Check sheet for the modelled part. Datum: model origin and axes. Units: mm. Coordinates: 2 decimals unless noted, no trailing zeros. Loops run counter-clockwise (first coordinate to the right, second up) from the corner with the lowest first, then second, coordinate; pieces in that order, holes last. Notation, with made-up numbers: (36.5, 20) - (69.5, 20) arc R17 cw to (69.5, 29) - close; hole circle Ø5 at (37.5, 38). An arc over 180 degrees is marked (long way). Write each question's results on one line, items separated by ' | '. Start each with the question number.
1. Cross-section at B-B (x = 2). Record the cut outline in (y, z).
2. Gauge pin test, flat ends, axial feed: P1, Ø1.5, axis at x = 30.5, y = 5.5, coming from the +Z side; P2, Ø0.9, axis at y = 31.5, z = 1, coming from the -X side. Record the tip position at first contact, or that the pin passes through.
3. Cross-section at A-A (y = 13). Record the cut outline in (x, z).
4. Thickness scan on line 1 (Y direction, x = 12.5, z = 0.5); line 2 (Y direction, x = 11, z = 0.2); line 3 (Y direction, x = 41, z = 1.3). Record the ranges inside material, lowest first. Write a range as [from, to].
```python
from build123d import *

# Parameters (mm, degrees)
F1_DEPTH = 1.524


with BuildPart() as f1:
    # F0 (on Top) → F1 (new body)
    with BuildSketch(Plane.XY):
        with BuildLine():
            ThreePointArc((-10.328003, 23.34511), (-10.546485, 19.972041), (-10.513837, 16.592061))
            Line((-10.513837, 16.592061), (10.397906, 16.369229))
            Line((10.397906, 16.369229), (10.397906, 16.592061))
            ThreePointArc((10.397906, 16.592061), (10.430555, 19.972041), (10.212073, 23.34511))
            ThreePointArc((10.212073, 23.34511), (9.373504, 27.05499), (8.504586, 30.75788))
            Line((8.504586, 30.75788), (8.504586, 31.872794))
            ThreePointArc((8.504586, 31.872794), (9.226054, 34.37206), (9.788919, 36.91175))
            ThreePointArc((9.788919, 36.91175), (9.766765, 38.207065), (9.636335, 39.495986))
            ThreePointArc((9.636335, 39.495986), (6.067855, 48.539888), (-0.057965, 56.089759))
            ThreePointArc((-0.057965, 56.089759), (-6.183786, 48.539888), (-9.752265, 39.495986))
            ThreePointArc((-9.752265, 39.495986), (-9.882696, 38.207065), (-9.904849, 36.91175))
            ThreePointArc((-9.904849, 36.91175), (-9.341984, 34.37206), (-8.620516, 31.872794))
            Line((-8.620516, 31.872794), (-8.620516, 30.75788))
            ThreePointArc((-8.620516, 30.75788), (-9.489434, 27.05499), (-10.328003, 23.34511))
        make_face()
        with BuildLine():
            ThreePointArc((-14.396, 23.613142), (-27.322804, 15.78758), (-27.740605, 0.682378))
            ThreePointArc((-27.740605, 0.682378), (-23.982132, 1.254002), (-20.641251, 3.06822))
            Line((-20.641251, 3.06822), (-19.369999, 0.811142))
            Line((-19.369999, 0.811142), (-9.112228, -17.40128))
            Line((-9.112228, -17.40128), (-7.869689, -19.607378))
            ThreePointArc((-7.869689, -19.607378), (-10.90344, -21.545267), (-13.251581, -24.273872))
            ThreePointArc((-13.251581, -24.273872), (-0.011043, -31.556032), (13.279346, -24.365258))
            ThreePointArc((13.279346, -24.365258), (10.905069, -21.396137), (7.663469, -19.409958))
            Line((7.663469, -19.409958), (8.978424, -17.187422))
            Line((8.978424, -17.187422), (19.626065, 0.809219))
            Line((19.626065, 0.809219), (20.915332, 2.988339))
            ThreePointArc((20.915332, 2.988339), (24.110468, 1.329978), (27.647581, 0.660731))
            ThreePointArc((27.647581, 0.660731), (27.333847, 15.768452), (14.461259, 23.68288))
            ThreePointArc((14.461259, 23.68288), (13.077063, 20.142135), (12.977783, 16.341738))
            Line((12.977783, 16.341738), (10.397906, 16.369229))
            Line((10.397906, 16.369229), (-10.513837, 16.592061))
            Line((-10.513837, 16.592061), (-13.045643, 16.61904))
            ThreePointArc((-13.045643, 16.61904), (-13.207029, 20.215289), (-14.396, 23.613142))
        make_face()
        with BuildLine():
            Line((-9.112228, -17.40128), (-19.369999, 0.811142))
            Line((-19.369999, 0.811142), (-19.5681, 0.708821))
            ThreePointArc((-19.5681, 0.708821), (-22.511572, -0.952895), (-25.323495, -2.828641))
            ThreePointArc((-25.323495, -2.828641), (-28.117061, -5.409803), (-30.889398, -8.013752))
            Line((-30.889398, -8.013752), (-31.854942, -8.571209))
            ThreePointArc((-31.854942, -8.571209), (-34.380104, -9.196033), (-36.860973, -9.978423))
            ThreePointArc((-36.860973, -9.978423), (-37.971671, -10.645265), (-39.022695, -11.402682))
            ThreePointArc((-39.022695, -11.402682), (-45.070704, -19.015027), (-48.546173, -28.095079))
            ThreePointArc((-48.546173, -28.095079), (-38.944884, -29.62526), (-29.328395, -28.193702))
            ThreePointArc((-29.328395, -28.193702), (-28.146941, -27.662198), (-27.014089, -27.033726))
            ThreePointArc((-27.014089, -27.033726), (-25.096085, -25.276425), (-23.292391, -23.401983))
            Line((-23.292391, -23.401983), (-22.326847, -22.844526))
            ThreePointArc((-22.326847, -22.844526), (-18.685592, -21.745586), (-15.053457, -20.616868))
            ThreePointArc((-15.053457, -20.616868), (-12.023052, -19.119545), (-9.112228, -17.40128))
        make_face()
        with BuildLine():
            Line((19.626065, 0.809219), (8.978424, -17.187422))
            Line((8.978424, -17.187422), (9.170193, -17.300882))
            ThreePointArc((9.170193, -17.300882), (12.081018, -19.019146), (15.111422, -20.51647))
            ThreePointArc((15.111422, -20.51647), (18.743557, -21.645188), (22.384812, -22.744127))
            Line((22.384812, -22.744127), (23.350356, -23.301585))
            ThreePointArc((23.350356, -23.301585), (25.15405, -25.176027), (27.072054, -26.933327))
            ThreePointArc((27.072054, -26.933327), (28.204906, -27.561799), (29.38636, -28.093304))
            ThreePointArc((29.38636, -28.093304), (39.002849, -29.524861), (48.604139, -27.99468))
            ThreePointArc((48.604139, -27.99468), (45.128669, -18.914629), (39.08066, -11.302284))
            ThreePointArc((39.08066, -11.302284), (38.029636, -10.544867), (36.918938, -9.878024))
            ThreePointArc((36.918938, -9.878024), (34.438069, -9.095634), (31.912908, -8.470811))
            Line((31.912908, -8.470811), (30.947364, -7.913354))
            ThreePointArc((30.947364, -7.913354), (28.175026, -5.309404), (25.38146, -2.728242))
            ThreePointArc((25.38146, -2.728242), (22.569538, -0.852496), (19.626065, 0.809219))
        make_face()
    extrude(amount=F1_DEPTH)


solid = f1.part
```
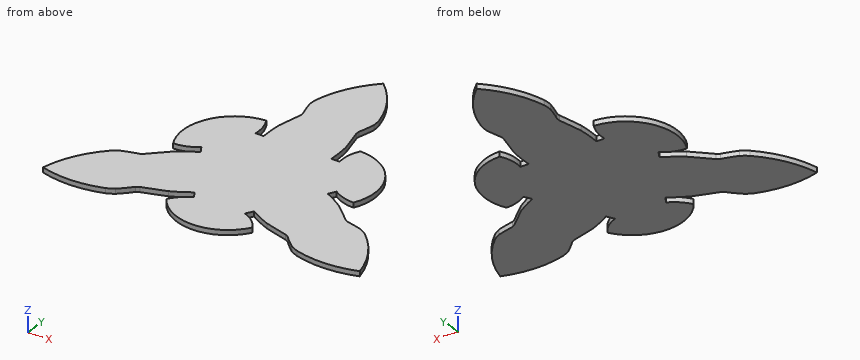
Established:
1) outline: (-31.43, 0) - (54.05, 0) - (54.05, 1.52) - (-31.43, 1.52) - close
2) P1: through | P2: x = -8.65
3) outline: (-28.6, 0) - (28.58, 0) - (28.58, 1.52) - (-28.6, 1.52) - close
4) line 1: [-25.46, -23.14], [-19.24, 16.35] | line 2: [-27.13, -21.48], [-18.41, 16.36] | line 3: [-29.45, -13.24]
